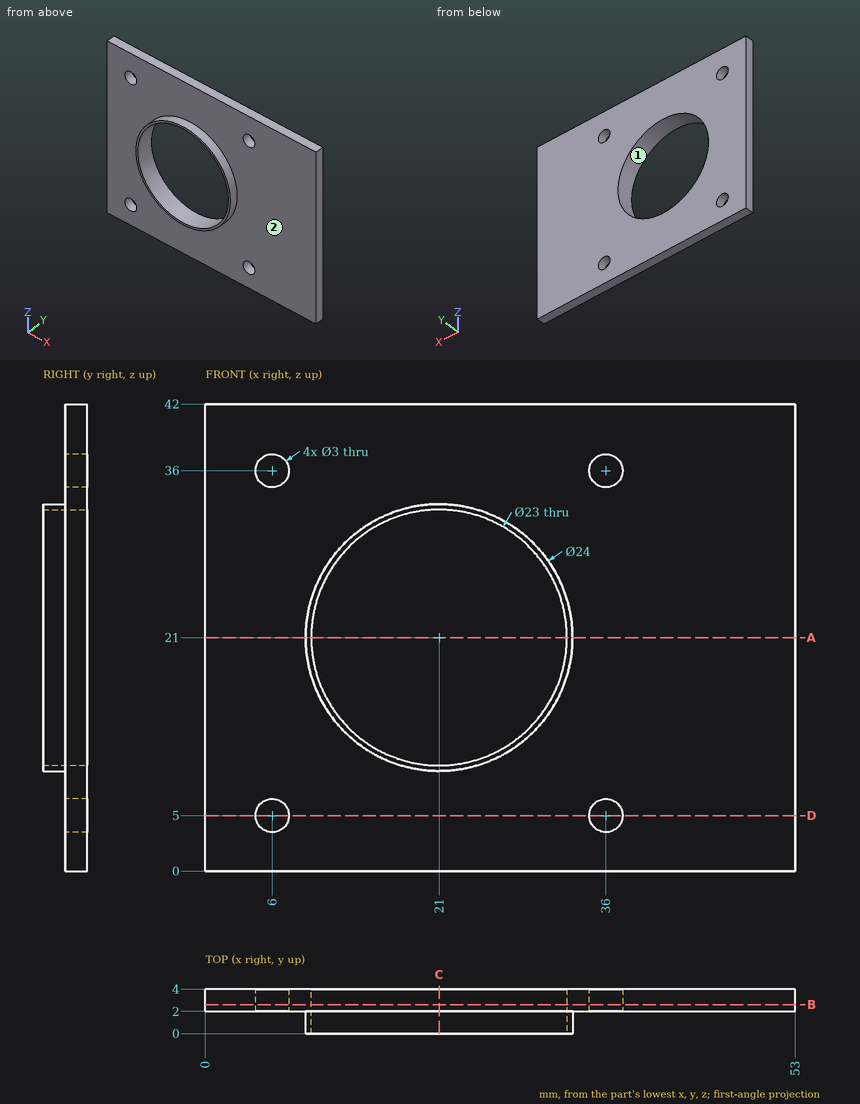
Source: three-view drawing plus pictorial views. Frame: mm from the lowest corner of the part. Coordinates: 2 decimals unless noted, no trailing zeros. Order: outer loops, then holes, each group sorted by start corner. A loop starts at its lowest first (then second) coordinate and runs counter-clockwise, first axis right, second up. Notation, with made-up numbers: M 23.25,62.25 L 71.25,62.25 A24 ccw 71.25,97.25 Z; hole C 37,-14 d11. An arc over 180 degrees is marked long. One line per question, with ' | ' between items.
Item 1: Section B-B (y = 2.6). Output: boundary loops of the cut face in (x, z), then the cut area to 3 significant figures.
Geometry results:
outline: M 0,0 L 53,0 L 53,42 L 0,42 Z; hole C 6,5 d3; hole C 6,36 d3; hole C 21,21 d23; hole C 36,5 d3; hole C 36,36 d3 | area: 1,780 mm^2
Item 2: Draft query along X for the marked faces 1 and 2. Return one class per face: released by +X, released by -X, zero draft, split by the parting line, or undercut.
Geometry results:
face 1: undercut | face 2: zero draft
Item 3: Ray query, line 1 along Z through (x, y) = (6, 3.55); line 2 along Z through (x, y) = (21, 1.25); line 3 along Y through (x, z) = (50.5, 24.5). Return the intervals inside material, ascending.
Geometry results:
line 1: z = 0 to 3.5, 6.5 to 34.5, 37.5 to 42 | line 2: z = 9 to 9.5, 32.5 to 33 | line 3: y = 2 to 4
Item 4: Section D-D (z = 5). Output: boundary loops of the cut face in (x, y).
Geometry results:
outline: M 0,2 L 4.5,2 L 4.5,4 L 0,4 Z; M 7.5,2 L 34.5,2 L 34.5,4 L 7.5,4 Z; M 37.5,2 L 53,2 L 53,4 L 37.5,4 Z
Item 5: Pin query (flat end, axial travel): pin 1 (14 mm diameter, centred on x = 21, z = 21, fed in from -Y); pin 2 (4 mm diameter, centred on x = 6, z = 36, fed in from -Y); pin 3 (1 mm diameter, centred on x = 11, y = 0.5, fed in from +Z). Return the tip coordinate at first contact, or that it passes through.
Geometry results:
pin 1: passes through | pin 2: stops at y = 2 | pin 3: stops at z = 28.33
Item 6: Section C-C (x = 21). Output: boundary loops of the cut face in (y, z), then the cut area to 3 significant figures.
Geometry results:
outline: M 0,9 L 2,9 L 2,0 L 4,0 L 4,9.5 L 0,9.5 Z; M 0,32.5 L 4,32.5 L 4,42 L 2,42 L 2,33 L 0,33 Z | area: 40.0 mm^2
Item 7: Section A-A (z = 21). Output: boundary loops of the cut face in (x, y), then the cut area to 3 significant figures.
Geometry results:
outline: M 0,2 L 9,2 L 9,0 L 9.5,0 L 9.5,4 L 0,4 Z; M 32.5,0 L 33,0 L 33,2 L 53,2 L 53,4 L 32.5,4 Z | area: 62.0 mm^2
